```python
from build123d import *

# Parameters (mm, degrees)
F0_W        = 127
F0_H        = 127
F1_DEPTH    = 203.2
F3_D        = 19.05
F4_SIZE     = 6.35
F5_T1_DEPTH = 210.0012806053
F5_T3_DEPTH = 146.05
F5_T5_DEPTH = 146.05
F6_R        = 5.08
F7_R        = 5.08
F9_DEPTH    = 76.2


# Not quite as in the source:
# - a fillet or chamfer that OpenCascade refuses, or shapes differently, is made with other operations: its cross-section is extruded or revolved along the edge and cut away or added


with BuildPart() as f1:
    # F0 (on Front) → F1 (new body)
    with BuildSketch(Plane.XZ):
        with Locations((63.5, 63.5)):
            Rectangle(F0_W, F0_H)
    extrude(amount=F1_DEPTH)

    # F3 (through all)
    with Locations(Plane.YZ.offset(127)):
        with Locations((-109.707146883, 106.2569767237), (-51.8769121036, 69.3713248935), (-112.7359410134, 37.7316983828)):
            Hole(F3_D / 2)

    # F4
    f4_edges = [f1.edges().sort_by_distance(p)[0] for p in [
        (63.5, -203.2, 127),
        (0, -203.2, 63.5),
        (127, -203.2, 63.5),
        (63.5, -203.2, 0),
        (127, -101.6, 0),
        (127, -101.6, 127),
        (0, -101.6, 127),
    ]]
    chamfer(f4_edges, length=F4_SIZE)

    # F5: fillet of radius 6.35 on 7 edges, made by hand

    # F5_s2 → F5_t1 (cut)
    with BuildSketch(Plane.XZ.offset(-6.5756403027)):
        with BuildLine():
            ThreePointArc((4.4901280605, 125.1401280605), (6.5502163256, 126.5166350314), (8.9802561211, 127))
            Line((8.9802561211, 127), (6.35, 127))
            Line((6.35, 127), (4.4901280605, 125.1401280605))
        make_face()
        with BuildLine():
            ThreePointArc((125.1401280605, 4.4901280605), (126.5166350314, 6.5502163256), (127, 8.9802561211))
            Line((127, 8.9802561211), (127, 6.35))
            Line((127, 6.35), (125.1401280605, 4.4901280605))
        make_face()
    extrude(amount=F5_T1_DEPTH, mode=Mode.SUBTRACT)

    # F5_s4 → F5_t3 (cut)
    with BuildSketch(Plane.YZ.offset(-9.525)):
        with BuildLine():
            ThreePointArc((0, 120.65), (-1.8598719395, 125.1401280605), (-6.35, 127))
            Line((-6.35, 127), (0, 127))
            Line((0, 127), (0, 120.65))
        make_face()
    extrude(amount=F5_T3_DEPTH, mode=Mode.SUBTRACT)

    # F5_s6 → F5_t5 (cut)
    with BuildSketch(Plane.XY.offset(-9.525)):
        with BuildLine():
            ThreePointArc((120.65, 0), (125.1401280605, -1.8598719395), (127, -6.35))
            Line((127, -6.35), (127, 0))
            Line((127, 0), (120.65, 0))
        make_face()
    extrude(amount=F5_T5_DEPTH, mode=Mode.SUBTRACT)

    # F5_s7 → F5_t8 (revolve, cut)
    with BuildSketch(Plane.XY.offset(106.2569767237)):
        with BuildLine():
            ThreePointArc((120.65, -100.182146883), (125.1401280605, -98.3222749435), (127, -93.832146883))
            Line((127, -93.832146883), (127, -100.182146883))
            Line((127, -100.182146883), (120.65, -100.182146883))
        make_face()
    revolve(axis=Axis((127, -109.707146883, 106.2569767237), (1, 0, 0)), mode=Mode.SUBTRACT)

    # F5_s9 → F5_t10 (revolve, cut)
    with BuildSketch(Plane.XY.offset(37.7316983828)):
        with BuildLine():
            ThreePointArc((120.65, -103.2109410134), (125.1401280605, -101.3510690739), (127, -96.8609410134))
            Line((127, -96.8609410134), (127, -103.2109410134))
            Line((127, -103.2109410134), (120.65, -103.2109410134))
        make_face()
    revolve(axis=Axis((127, -112.7359410134, 37.7316983828), (1, 0, 0)), mode=Mode.SUBTRACT)

    # F5_s11 → F5_t12 (revolve, cut)
    with BuildSketch(Plane.XY.offset(69.3713248935)):
        with BuildLine():
            ThreePointArc((120.65, -42.3519121036), (125.1401280605, -40.4920401641), (127, -36.0019121036))
            Line((127, -36.0019121036), (127, -42.3519121036))
            Line((127, -42.3519121036), (120.65, -42.3519121036))
        make_face()
    revolve(axis=Axis((127, -51.8769121036, 69.3713248935), (1, 0, 0)), mode=Mode.SUBTRACT)

    # F6
    f6_edges = [f1.edges().sort_by_distance(p)[0] for p in [
        (6.35, -203.2, 63.5),
        (63.5, -203.2, 6.35),
    ]]
    fillet(f6_edges, radius=F6_R)

    # F7
    f7_edges = [f1.edges().sort_by_distance(p)[0] for p in [
        (60.325, 0, 0),
        (0, 0, 60.325),
    ]]
    fillet(f7_edges, radius=F7_R)

    # F8 (on face) → F9 (join)
    with BuildSketch(Plane(origin=(0, 0, 0), x_dir=(-1, 0, 0), z_dir=(0, 1, 0))):
        Polygon((-100.4286549397, 40.3320468052), (-120.65, 5.08), (-54.4255593013, 5.08), (-54.4255593013, 9.1751408411), (-75.2091502909, 31.4702691336), (-64.1732869808, 55.1769325335), (-86.5088332529, 75.9170813451), (-118.2750036349, 50.5691027419), align=None)
    extrude(amount=F9_DEPTH)


solid = f1.part
```
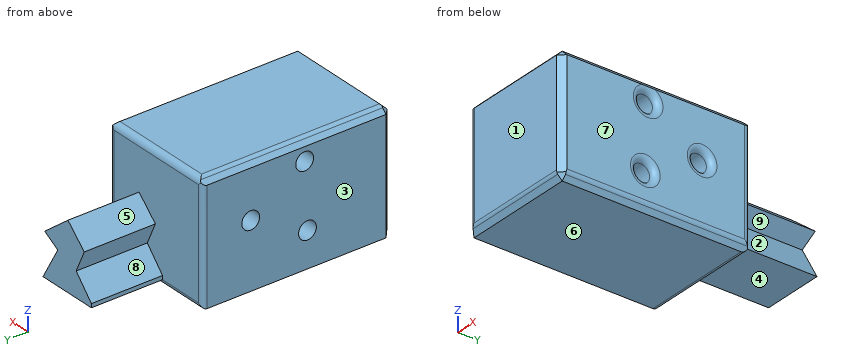
Could you check a few things on this model? Use its own coordinates, in mm. Face numbers are marked on the shaded views. A direction names the side the tool comes from. Coordinates: 2 decimals unless noted, no trailing zeros. Write each loop counter-clockwise with the first axis right and the second up, starting at its lowest first coordinate (ties: lowest second). Pieces come first, ordered by that corner, then holes. Notation, with made-up numbers: M 23.25,24 L 64.25,24 A24 cw 64.25,48 Z; hole C 36,-38.75 d1. An arc over 180 degrees is marked long. Answer as CSV lines item,"result". Start each with the question number.
1) We'd pull the mould along Z, two halves only. Please class the marked faces 6, 7, 8 and 9: +Z half, -Z half, draft (parallel to the pull), parting line (faces both ways), or undercut.
2) I want a section at D-D, the plane x = 38. Please give me the cut outline in (y, z) (3 decimals), and give its area (3 significant figures).
3) Please list where these lines run through material, in increasing order: line 1 (Y direction, x = 95, z = 33); line 2 (Y direction, x = 7, z = 69.5); line 3 (Y direction, x = 17.5, z = 13). Write a range as from..to.
4) I want a section at A-A, the plane y = 11.5. Please give me the cut outline in (x, z) (3 decimals), and give its area (3 significant figures).
5) I want a section at C-C, the plane z = 15.5. Please give me the cut outline in (x, y), and give its area (3 significant figures).
6) I want a section at B-B, the plane x = 59.5. Please give me the cut outline in (y, z) (3 decimals), and give its area (3 significant figures).
7) For the marked faces 1, 2, 3, 4 and 5, which set-ups out of +Z, -Z, +X, -X, +Y, -Y let a thin tool reach every point of the face, with its end or its side?
8) For P1, Ø4.5, axis at y = 26, z = 6.5, coming from the -X side; P2, Ø10, axis at x = 100.5, y = 33.5, coming from the -Z side; P3, Ø8, axis at x = 15, z = 47, coming from the +Y side, each with a flat end and sliding along its axis, tell me the tip position at first contact or that it passes through.
Data:
1,face 6,"-Z half"
1,face 7,"draft"
1,face 8,"undercut"
1,face 9,"undercut"
2,outline,"M -203.2,8.454 A5.08 ccw -201.712,4.862 L -196.85,0 L -5.08,0 A5.08 ccw 0,5.08 L 0,120.65 A6.35 ccw -6.35,127 L -196.85,127 L -203.2,120.65 Z; hole C -112.736,37.732 d19.05; hole C -109.707,106.257 d19.05; hole C -51.877,69.371 d19.05"
2,area,"24,900 mm^2"
3,line 1,"y = -203.2..-121, -104.47..76.2"
3,line 2,"y = -202.99..-61.4, -42.35..0"
3,line 3,"y = -203.2..0"
4,outline,"M 54.426,5.08 L 120.65,5.08 L 100.429,40.332 L 118.275,50.569 L 86.509,75.917 L 64.173,55.177 L 75.209,31.47 L 54.426,9.175 Z"
4,area,"2,730 mm^2"
5,outline,"M 0,-196.85 L 4.86,-201.71 A5.08 ccw 8.45,-203.2 L 120.65,-203.2 L 127,-196.85 L 127,-6.35 A6.35 ccw 120.65,0 L 114.67,0 L 114.67,76.2 L 60.32,76.2 L 60.32,0 L 5.08,0 A5.08 ccw 0,-5.08 Z"
5,area,"29,900 mm^2"
6,outline,"M -203.2,8.454 A5.08 ccw -201.712,4.862 L -196.85,0 L -5.08,0 A5.08 ccw 0,5.08 L 76.2,5.08 L 76.2,14.619 L 0,14.619 L 0,120.65 A6.35 ccw -6.35,127 L -196.85,127 L -203.2,120.65 Z; hole C -112.736,37.732 d19.05; hole C -109.707,106.257 d19.05; hole C -51.877,69.371 d19.05"
6,area,"25,600 mm^2"
7,face 1,"+Z, -Z, +X, -X, -Y"
7,face 2,"+X, +Y"
7,face 3,"+Z, -Z, -X, +Y, -Y"
7,face 4,"-Z, +X, -X, +Y"
7,face 5,"+Z, -X, +Y"
8,P1,"stops at x = 54.43"
8,P2,"stops at z = 5.08"
8,P3,"stops at y = 0"
